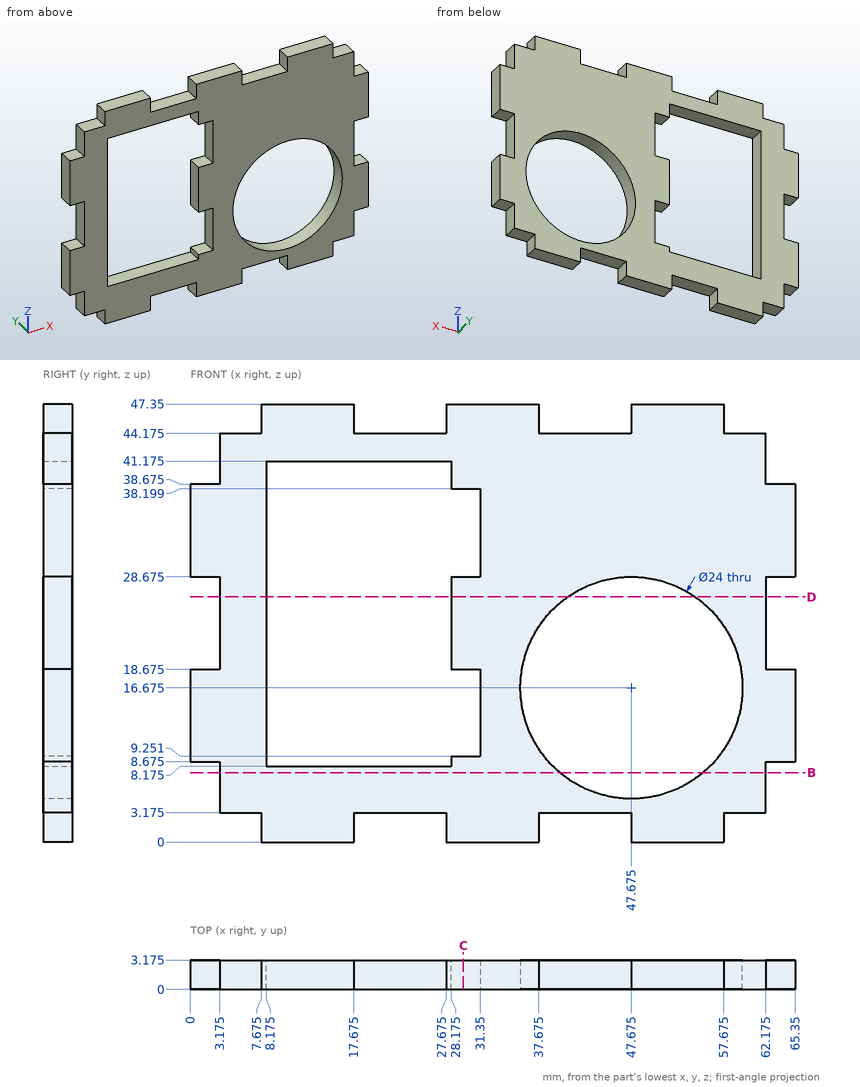
The figure shows three views and two pictorial views of one solid part (mm, origin at its lowest corner). Answer the questions. Round coordinates to 2 decimals unless told otherwise and drop trailing zeros. Loops run counter-clockwise (first coordinate to the right, second up) from the corner with the lowest first, then second, coordinate; pieces in that order, holes last. Notation, with made-up numbers: (39, 22.5) - (79, 22.5) arc R31 cw to (79, 56.5) - close; hole circle Ø8 at (-14, 5.25). An arc over 180 degrees is marked (long way). Use one line per item in the form item = value. Start each with the question number.
(1) Find section C-C on x = 29.5. Give the number of separate pieces and of enclosed holes in the cut face.
(2) Find section B-B on z = 7.5. Determine the outline of the cut face in (x, y) (1 decimal).
(3) Find section D-D on z = 26.5. Determine the outline of the cut face in (x, y) (1 decimal).
(4) Consider line 1 (Z direction, x = 27, y = 0.3) (1 decimal); line 2 (Z direction, x = 45, y = 0.7) (1 decimal); line 3 (Z direction, x = 5, y = 2.6) (1 decimal). Determine where each line is inside the solid, lowest interval first.
(5) Flat-ended cylindrical pins translate along their axes: P1, Ø1, axis at x = 2, y = 2, coming from the +Z side (3 decimals); P2, Ø1.6, axis at y = 2, z = 7, coming from the -X side (3 decimals); P3, Ø1, axis at x = 24, y = 2, coming from the +Z side (3 decimals); P4, Ø1, axis at x = 30.5, y = 1.5, coming from the -Z side. Find the tip coordinate at first contact, or state that the pin passes through.
Answer list:
q1.separate_pieces = 3
q1.enclosed_holes = 0
q2.outline = (3.2, 0) - (39.9, 0) - (39.9, 3.2) - (3.2, 3.2) - close; (55.4, 0) - (62.2, 0) - (62.2, 3.2) - (55.4, 3.2) - close
q3.outline = (3.2, 0) - (8.2, 0) - (8.2, 3.2) - (3.2, 3.2) - close; (28.2, 0) - (40.8, 0) - (40.8, 3.2) - (28.2, 3.2) - close; (54.6, 0) - (62.2, 0) - (62.2, 3.2) - (54.6, 3.2) - close
q4.line_1 = 3.2 to 8.2, 41.2 to 44.2
q4.line_2 = 3.2 to 5, 28.4 to 44.2
q4.line_3 = 3.2 to 44.2
q5.P1 = 38.675
q5.P2 = 3.175
q5.P3 = 44.175
q5.P4 = 0
